Verification items for the finished model (mm, model axes). A direction names the side the tool comes from. Round coordinates to 2 decimals unless told otherwise and drop trailing zeros. Order: outer loops, then holes, each group sorted by start corner. A loop starts at its lowest first (then second) coordinate and runs counter-clockwise, first axis right, second up. Notation, with made-up numbers: M 86,37 L 142,37 A15 cw 142,64 Z; hole C 58,-19 d3. An arc over 180 degrees is marked long. Return JSON: item names as keys, results as strings. Group by question number.
from build123d import *

# Parameters (mm, degrees)
SKETCH1_W      = 50
SKETCH1_H      = 50
SKETCH1_R      = 1.5
SKETCH1_R_2    = 1.646935024
SKETCH1_R_3    = 1.908192471
SKETCH1_R_4    = 1.759080553
EXTRUDE2_DEPTH = 0.8
SKETCH2_W      = 6
SKETCH2_H      = 12.5
EXTRUDE3_DEPTH = 7
SKETCH3_W      = 6
SKETCH3_H      = 12.5
EXTRUDE4_DEPTH = 7
SKETCH4_W      = 39
SKETCH4_H      = 23
EXTRUDE5_DEPTH = 8.5
SKETCH5_R      = 2.5
EXTRUDE8_DEPTH = 11


with BuildPart() as part:
    # Sketch1 → Extrude2 (new, symmetric)
    with BuildSketch(Plane.XY):
        Rectangle(SKETCH1_W, SKETCH1_H)
        with Locations((-22, 22)):
            Circle(SKETCH1_R, mode=Mode.SUBTRACT)
        with Locations((22, 22)):
            Circle(SKETCH1_R_2, mode=Mode.SUBTRACT)
        with Locations((22, -22)):
            Circle(SKETCH1_R_3, mode=Mode.SUBTRACT)
        with Locations((-22, -22)):
            Circle(SKETCH1_R_4, mode=Mode.SUBTRACT)
    extrude(amount=EXTRUDE2_DEPTH, both=True)

    # Sketch2 → Extrude3 (add)
    with BuildSketch(Plane.XY.offset(0.8)):
        with Locations((7, 12.25)):
            Rectangle(SKETCH2_W, SKETCH2_H)
        with Locations((7, -12.25)):
            Rectangle(SKETCH2_W, SKETCH2_H)
        with Locations((0.7, 12.25)):
            Rectangle(SKETCH2_W, SKETCH2_H)
        with Locations((0.7, -12.25)):
            Rectangle(SKETCH2_W, SKETCH2_H)
        with Locations((-5.6, 12.25)):
            Rectangle(SKETCH2_W, SKETCH2_H)
        with Locations((-5.6, -12.25)):
            Rectangle(SKETCH2_W, SKETCH2_H)
    extrude(amount=EXTRUDE3_DEPTH)

    # Sketch3 → Extrude4 (add)
    with BuildSketch(Plane(origin=(0, 0, -0.8), x_dir=(-1, 0, 0), z_dir=(0, 0, -1))):
        with Locations((-22.5, -6.25)):
            Rectangle(SKETCH3_W, SKETCH3_H)
    extrude(amount=EXTRUDE4_DEPTH)

    # Sketch4 → Extrude5 (add)
    with BuildSketch(Plane(origin=(0, 0, -0.8), x_dir=(-1, 0, 0), z_dir=(0, 0, -1))):
        with Locations((0, -13)):
            Rectangle(SKETCH4_W, SKETCH4_H)
        with Locations((0, 13)):
            Rectangle(SKETCH4_W, SKETCH4_H)
    extrude(amount=EXTRUDE5_DEPTH)

    # Sketch5 → Extrude8 (add)
    with BuildSketch(Plane(origin=(0, 0, -0.8), x_dir=(-1, 0, 0), z_dir=(0, 0, -1))):
        with Locations(Location((22.4, -3, 0), (0, 0, 180))):
            Circle(SKETCH5_R)
        with Locations(Location((22.4, 3, 0), (0, 0, 180))):
            Circle(SKETCH5_R)
        with Locations(Location((-22.4, -15.2, 0), (0, 0, 180))):
            Circle(SKETCH5_R)
        with Locations(Location((-22.4, 4, 0), (0, 0, 180))):
            Circle(SKETCH5_R)
    extrude(amount=EXTRUDE8_DEPTH)


solid = part.part
1. Draft check along Y on faces 6 (the face through (0, -24.5, -5)), 7 (the face through (-22, -3, -11.8)), 8 (the face through (-6, -6, 4)). Enter one of: +Y half, -Y half, draft (parallel to the pull), parting line (faces both ways), or undercut.
2. Access from +Z, -Z, +X, -X, +Y, -Y to the whole of each face (thin tool, end or side, straight path). Record for faces 1 (the face through (-6, 18.5, 4)), 2 (the face through (0, -13, -9.3)), 3 (the face through (10, -12, 4)), 4 (the face through (1, -18.5, 4)), 5 (the face through (-2.6, 12, 4)).
3. Cross-section at C-C (x = 12). Enter the section's corners in (y, z), plus the area to 3 significant figures.
4. Go/stop test with flat-tipped pins: pin 1 (3 mm diameter, centred on x = -5, z = 4.5, fed in from +Y); pin 2 (3 mm diameter, centred on x = -5, z = 4.5, fed in from -Y); pin 3 (2 mm diameter, centred on y = -12, z = 3.5, fed in from -X). Record where each tip stops, or that it passes through.
5. Thickness scan on line 1 along Y through (x, z) = (-22, -0.4); line 2 along Y through (x, z) = (22, -0.4); line 3 along Y through (x, z) = (19, -2.5). Record the ranges inside material, lowest first. Write a range as from..to.
6. Cross-section at B-B (y = 22). Enter the section's corners in (x, z).
7. Cross-section at D-D (y = 9.5). Enter the section's corners in (x, z), plus the area to 4 significant figures.
8. Cross-section at A-A (z = -6). Enter the section's corners in (x, y), plus the area to 3 significant figures.
Computed:
{
 "1": {"face 6": "-Y half", "face 7": "draft", "face 8": "undercut"},
 "2": {"face 1": "+Z, +X, -X, +Y", "face 2": "-Z, +Y, -Y", "face 3": "+Z, +X, +Y, -Y", "face 4": "+Z, +X, -X, -Y", "face 5": "+Z, +Y, -Y"},
 "3": {"outline": "M -25,-0.8 L -24.5,-0.8 L -24.5,-9.3 L -1.5,-9.3 L -1.5,-0.8 L 1.5,-0.8 L 1.5,-9.3 L 24.5,-9.3 L 24.5,-0.8 L 25,-0.8 L 25,0.8 L -25,0.8 Z", "area": "471 mm²"},
 "4": {"pin 1": "stops at y = 18.5", "pin 2": "stops at y = -18.5", "pin 3": "stops at x = -8.6"},
 "5": {"line 1": "y = -25..-23.76, -20.24..20.5, 23.5..25", "line 2": "y = -25..-23.91, -20.09..20.35, 23.65..25", "line 3": "y = -24.5..-1.5, 1.5..24.5"},
 "6": {"outline": "M -25,-0.8 L -23.5,-0.8 L -23.5,0.8 L -25,0.8 Z; M -20.5,-0.8 L -19.5,-0.8 L -19.5,-9.3 L 19.5,-9.3 L 19.5,-0.8 L 20.35,-0.8 L 20.35,0.8 L -20.5,0.8 Z; M 23.65,-0.8 L 25,-0.8 L 25,0.8 L 23.65,0.8 Z"},
 "7": {"outline": "M -25,-0.8 L -19.5,-0.8 L -19.5,-9.3 L 19.5,-9.3 L 19.5,-0.8 L 25,-0.8 L 25,0.8 L 10,0.8 L 10,7.8 L 4,7.8 L 4,0.8 L 3.7,0.8 L 3.7,7.8 L -2.3,7.8 L -2.3,0.8 L -2.6,0.8 L -2.6,7.8 L -8.6,7.8 L -8.6,0.8 L -25,0.8 Z", "area": "537.5 mm²"},
 "8": {"outline": "C -22.4,-3 d5; C -22.4,3 d5; M -19.5,-24.5 L 19.5,-24.5 L 19.5,-12.5 L 25.5,-12.5 L 25.5,0 L 19.5,0 L 19.5,-1.5 L -19.5,-1.5 Z; M -19.5,1.5 L 19.5,1.5 L 19.5,24.5 L -19.5,24.5 Z; C 22.4,-15.2 d5; C 22.4,4 d5", "area": "1,950 mm²"}
}
